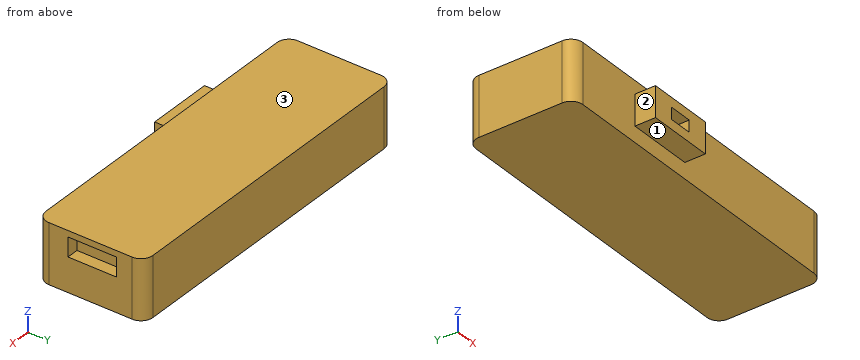
```python
from build123d import *

# Parameters (mm, degrees)
BOSS_EXTRUDE1_DEPTH = 12.7
SKETCH2_W           = 4.090641248
SKETCH2_H           = 10.364450922
CUT_EXTRUDE1_DEPTH  = 2.54
SKETCH3_W           = 14.14
SKETCH3_H           = 6.54
SKETCH3_W_2         = 5.008
SKETCH3_H_2         = 2.508
BOSS_EXTRUDE2_DEPTH = 4.39457265


with BuildPart() as part:
    # Sketch1 → Boss-Extrude1 (new body)
    with BuildSketch(Plane.XY):
        with BuildLine():
            Line((-19.05, 11.43), (46.542212097, 11.43))
            ThreePointArc((46.542212097, 11.43), (48.338263321, 10.686051224), (49.082212097, 8.89))
            Line((49.082212097, 8.89), (49.082212097, -8.89))
            ThreePointArc((49.082212097, -8.89), (48.338263321, -10.686051224), (46.542212097, -11.43))
            Line((46.542212097, -11.43), (-19.05, -11.43))
            ThreePointArc((-19.05, -11.43), (-20.846051224, -10.686051224), (-21.59, -8.89))
            Line((-21.59, -8.89), (-21.59, 8.89))
            ThreePointArc((-21.59, 8.89), (-20.846051224, 10.686051224), (-19.05, 11.43))
        make_face()
    extrude(amount=-BOSS_EXTRUDE1_DEPTH)

    # Sketch2 → Cut-Extrude1 (cut)
    with BuildSketch(Plane(origin=(49.082212097, 0, 0), x_dir=(0, 0, -1), z_dir=(1, 0, 0))):
        with Locations((3.362716068, 0.383061409)):
            Rectangle(SKETCH2_W, SKETCH2_H)
    extrude(amount=-CUT_EXTRUDE1_DEPTH, mode=Mode.SUBTRACT)

    # Sketch3 → Boss-Extrude2 (add)
    with BuildSketch(Plane.XZ.offset(11.43)):
        with Locations((2.794, -6.064)):
            Rectangle(SKETCH3_W, SKETCH3_H)
        with Locations((2.794, -6.064)):
            Rectangle(SKETCH3_W_2, SKETCH3_H_2, mode=Mode.SUBTRACT)
    extrude(amount=BOSS_EXTRUDE2_DEPTH)


solid = part.part
```
The model under review builds one solid part; all positions refer to its coordinate system, in mm. Face numbers are marked on the shaded views. A direction names the side the tool comes from. Coordinates: 2 decimals unless noted, no trailing zeros. Order: outer loops, then holes, each group sorted by start corner. A loop starts at its lowest first (then second) coordinate and runs counter-clockwise, first axis right, second up. Notation, with made-up numbers: M 84,38.5 L 121,38.5 A30 cw 121,65.5 Z; hole C 67,-13 d5. An arc over 180 degrees is marked long. One line per question, with ' | ' between items.
(1) Add section C-C, the plane x = 2. Write out the cut boundary in (y, z), then the cut area to 3 significant figures.
Geometry results:
outline: M -15.82,-9.33 L -11.43,-9.33 L -11.43,-12.7 L 11.43,-12.7 L 11.43,0 L -11.43,0 L -11.43,-2.79 L -15.82,-2.79 L -15.82,-4.81 L -11.43,-4.81 L -11.43,-7.32 L -15.82,-7.32 Z | area: 308 mm²
(2) For probe 1 along Z at (x, y) = (0.5, -13.75); probe 2 along Y at (x, z) = (5, -7); probe 3 along X at (y, z) = (1, -2), list the stretches that pass through material, from the lowest coordinate up. Write a range as from..to.
Geometry results:
probe 1: z = -9.33..-7.32, -4.81..-2.79 | probe 2: y = -11.43..11.43 | probe 3: x = -21.59..46.54
(3) Machinability: for the marked faces 1, 2 and 3, which of the approach directions +Z, -Z, +X, -X, +Y, -Y give a long, thin tool a straight path to every point of the face, cutting with its end or side? Answer none if there is none.
Geometry results:
face 1: -Z, +X, -X, -Y | face 2: +Z, -Z, -X, -Y | face 3: +Z, +X, -X, +Y, -Y
(4) Insertion check: pin 1 (1.5 mm diameter, centred on x = 12, y = 1.5, fed in from +Z); pin 2 (1.3 mm diameter, centred on x = 3, y = -14, fed in from -Z); pin 3 (6.5 mm diameter, centred on x = 17, z = -5.5, fed in from -Y); pin 4 (5 mm diameter, centred on x = 3.5, y = -14, fed in from +Z). Each pin has a flat end and moves straight along its axis. Give the tip position at first contact, or say it passes through.
Geometry results:
pin 1: stops at z = 0 | pin 2: stops at z = -9.33 | pin 3: stops at y = -11.43 | pin 4: stops at z = -2.79
(5) Add section D-D, the plane z = -10.5. Write out the cut boundary in (x, y), then the cut area to 3 significant figures.
Geometry results:
outline: M -21.59,-8.89 A2.54 ccw -19.05,-11.43 L 46.54,-11.43 A2.54 ccw 49.08,-8.89 L 49.08,8.89 A2.54 ccw 46.54,11.43 L -19.05,11.43 A2.54 ccw -21.59,8.89 Z | area: 1,610 mm²
(6) Add section A-A, the plane z = -2. Write out the cut boundary in (x, y), then the cut area to 3 significant figures.
Geometry results:
outline: M -21.59,-8.89 A2.54 ccw -19.05,-11.43 L 46.54,-11.43 A2.54 ccw 49.08,-8.89 L 49.08,-4.8 L 46.54,-4.8 L 46.54,5.57 L 49.08,5.57 L 49.08,8.89 A2.54 ccw 46.54,11.43 L -19.05,11.43 A2.54 ccw -21.59,8.89 Z | area: 1,580 mm²
(7) Add section B-B, the plane y = -12.75. Write out the cut boundary in (x, z), then the cut area to 3 significant figures.
Geometry results:
outline: M -4.28,-9.33 L 9.86,-9.33 L 9.86,-2.79 L -4.28,-2.79 Z; hole M 0.29,-7.32 L 5.3,-7.32 L 5.3,-4.81 L 0.29,-4.81 Z | area: 79.9 mm²
